from build123d import *

# Parameters (mm, degrees)
SKETCH1_R                       = 57.15
BOSS_EXTRUDE1_DEPTH             = 201.2442
SKETCH3_W                       = 1.27
SKETCH3_H                       = 1.27
SKETCH9_R                       = 61.1124
BOSS_EXTRUDE4_DEPTH             = 6.35
SKETCH10_R                      = 61.1124
BOSS_EXTRUDE5_DEPTH             = 6.35
F_97_0_164_DIAMETER_HOLE1_D     = 4.1656
F_97_0_164_DIAMETER_HOLE1_DEPTH = 8.255
F_97_0_164_DIAMETER_HOLE1_TIP   = 1.251472497
F_97_0_352_DIAMETER_HOLE1_D     = 8.9408
CUT_EXTRUDE3_DEPTH              = 202.2442
SKETCH20_R                      = 49.53
CUT_EXTRUDE4_DEPTH              = 191.7192
FILLET4_R                       = 0.508
FILLET5_R                       = 0.254
CHAMFER1_SIZE                   = 0.762
CHAMFER2_SIZE                   = 1.6002


with BuildPart() as part:
    # Sketch1 → Boss-Extrude1 (new body)
    with BuildSketch(Plane.XY):
        Circle(SKETCH1_R)
    extrude(amount=BOSS_EXTRUDE1_DEPTH)

    # Sketch3 → Cut-Revolve2 (revolve, cut)
    with BuildSketch(Plane(origin=(0, 0, 0), x_dir=(0, 0, -1), z_dir=(1, 0, 0))):
        with Locations((-31.115, 56.515)):
            Rectangle(SKETCH3_W, SKETCH3_H)
        with Locations((-189.357, 56.515)):
            Rectangle(SKETCH3_W, SKETCH3_H)
    revolve(axis=Axis((0, 0, 212.826037786), (0, 0, -1)), mode=Mode.SUBTRACT)

    # Sketch9 → Boss-Extrude4 (add)
    with BuildSketch(Plane.XY.offset(188.722)):
        Circle(SKETCH9_R)
    extrude(amount=-BOSS_EXTRUDE4_DEPTH)

    # Sketch10 → Boss-Extrude5 (add)
    with BuildSketch(Plane(origin=(0, 0, 31.75), x_dir=(-1, 0, 0), z_dir=(0, 0, -1))):
        Circle(SKETCH10_R)
    extrude(amount=-BOSS_EXTRUDE5_DEPTH)

    # #97 (0.164) Diameter Hole1
    with Locations(Plane.XY.offset(201.2442)):
        with Locations((0, 53.34), (46.193795038, 26.67), (46.193795038, -26.67), (0, -53.34), (-46.193795038, -26.67), (-46.193795038, 26.67)):
            Hole(F_97_0_164_DIAMETER_HOLE1_D / 2, depth=F_97_0_164_DIAMETER_HOLE1_DEPTH)
            with Locations((0, 0, -(F_97_0_164_DIAMETER_HOLE1_DEPTH + F_97_0_164_DIAMETER_HOLE1_TIP / 2))):  # 118° drill point
                Cone(0, F_97_0_164_DIAMETER_HOLE1_D / 2, F_97_0_164_DIAMETER_HOLE1_TIP, mode=Mode.SUBTRACT)

    # #97 (0.352) Diameter Hole1 (through all)
    with Locations(Plane.XY.offset(201.2442)):
        with Locations((0, 38.735), (33.545494016, 19.3675), (33.545494016, -19.3675), (0, -38.735), (-33.545494016, -19.3675), (-33.545494016, 19.3675)):
            Hole(F_97_0_352_DIAMETER_HOLE1_D / 2)

    # Sketch18 → Cut-Extrude3 (cut, through all)
    with BuildSketch(Plane.XY.offset(201.2442)):
        with BuildLine():
            Line((26.579810552, 10.4902), (32.11926165, 10.4902))
            ThreePointArc((32.11926165, 10.4902), (36.312562564, 8.908714176), (38.417156092, 4.952003922))
            ThreePointArc((38.417156092, 4.952003922), (38.655457352, 2.481096914), (38.735, 0))
            ThreePointArc((38.735, 0), (38.655457352, -2.481096914), (38.417156092, -4.952003922))
            ThreePointArc((38.417156092, -4.952003922), (36.312562564, -8.908714176), (32.11926165, -10.4902))
            Line((32.11926165, -10.4902), (26.579810552, -10.4902))
            ThreePointArc((26.579810552, -10.4902), (24.746675913, -14.2875), (22.374684967, -17.773691165))
            Line((22.374684967, -17.773691165), (25.144410516, -22.57099654))
            ThreePointArc((25.144410516, -22.57099654), (25.871454074, -26.993244568), (23.497139241, -30.794231156))
            ThreePointArc((23.497139241, -30.794231156), (21.476421633, -32.236059605), (19.3675, -33.545494016))
            ThreePointArc((19.3675, -33.545494016), (17.179035719, -34.717156519), (14.92001685, -35.746235077))
            ThreePointArc((14.92001685, -35.746235077), (10.44110849, -35.901958745), (6.974851134, -33.06119654))
            Line((6.974851134, -33.06119654), (4.205125585, -28.263891165))
            ThreePointArc((4.205125585, -28.263891165), (0, -28.575), (-4.205125585, -28.263891165))
            Line((-4.205125585, -28.263891165), (-6.974851134, -33.06119654))
            ThreePointArc((-6.974851134, -33.06119654), (-10.44110849, -35.901958745), (-14.92001685, -35.746235077))
            ThreePointArc((-14.92001685, -35.746235077), (-17.179035719, -34.717156519), (-19.3675, -33.545494016))
            ThreePointArc((-19.3675, -33.545494016), (-21.476421633, -32.236059605), (-23.497139241, -30.794231156))
            ThreePointArc((-23.497139241, -30.794231156), (-25.871454074, -26.993244568), (-25.144410516, -22.57099654))
            Line((-25.144410516, -22.57099654), (-22.374684967, -17.773691165))
            ThreePointArc((-22.374684967, -17.773691165), (-24.746675913, -14.2875), (-26.579810552, -10.4902))
            Line((-26.579810552, -10.4902), (-32.11926165, -10.4902))
            ThreePointArc((-32.11926165, -10.4902), (-36.312562564, -8.908714176), (-38.417156092, -4.952003922))
            ThreePointArc((-38.417156092, -4.952003922), (-38.655457352, -2.481096914), (-38.735, 0))
            ThreePointArc((-38.735, 0), (-38.655457352, 2.481096914), (-38.417156092, 4.952003922))
            ThreePointArc((-38.417156092, 4.952003922), (-36.312562564, 8.908714176), (-32.11926165, 10.4902))
            Line((-32.11926165, 10.4902), (-26.579810552, 10.4902))
            ThreePointArc((-26.579810552, 10.4902), (-24.746675913, 14.2875), (-22.374684967, 17.773691165))
            Line((-22.374684967, 17.773691165), (-25.144410516, 22.57099654))
            ThreePointArc((-25.144410516, 22.57099654), (-25.871454074, 26.993244568), (-23.497139241, 30.794231156))
            ThreePointArc((-23.497139241, 30.794231156), (-21.476421633, 32.236059605), (-19.3675, 33.545494016))
            ThreePointArc((-19.3675, 33.545494016), (-17.179035719, 34.717156519), (-14.92001685, 35.746235077))
            ThreePointArc((-14.92001685, 35.746235077), (-10.44110849, 35.901958745), (-6.974851134, 33.06119654))
            Line((-6.974851134, 33.06119654), (-4.205125585, 28.263891165))
            ThreePointArc((-4.205125585, 28.263891165), (0, 28.575), (4.205125585, 28.263891165))
            Line((4.205125585, 28.263891165), (6.974851134, 33.06119654))
            ThreePointArc((6.974851134, 33.06119654), (10.44110849, 35.901958745), (14.92001685, 35.746235077))
            ThreePointArc((14.92001685, 35.746235077), (17.179035719, 34.717156519), (19.3675, 33.545494016))
            ThreePointArc((19.3675, 33.545494016), (21.476421633, 32.236059605), (23.497139241, 30.794231156))
            ThreePointArc((23.497139241, 30.794231156), (25.871454074, 26.993244568), (25.144410516, 22.57099654))
            Line((25.144410516, 22.57099654), (22.374684967, 17.773691165))
            ThreePointArc((22.374684967, 17.773691165), (24.746675913, 14.2875), (26.579810552, 10.4902))
        make_face()
    extrude(amount=-CUT_EXTRUDE3_DEPTH, mode=Mode.SUBTRACT)

    # Sketch20 → Cut-Extrude4 (cut)
    with BuildSketch(Plane.XY.offset(201.2442)):
        Circle(SKETCH20_R)
    extrude(amount=-CUT_EXTRUDE4_DEPTH, mode=Mode.SUBTRACT)

    # Fillet4
    fillet4_edges = [part.edges().sort_by_distance(p)[0] for p in [
        (-49.53, 0, 9.525),
    ]]
    fillet(fillet4_edges, radius=FILLET4_R)

    # Fillet5
    fillet5_edges = [part.edges().sort_by_distance(p)[0] for p in [
        (-57.15, 0, 182.372),
        (-57.15, 0, 38.1),
    ]]
    fillet(fillet5_edges, radius=FILLET5_R)

    # Chamfer1
    chamfer1_edges = [part.edges().sort_by_distance(p)[0] for p in [
        (-57.15, 0, 201.2442),
    ]]
    chamfer(chamfer1_edges, length=CHAMFER1_SIZE)

    # Chamfer2
    chamfer2_edges = [part.edges().sort_by_distance(p)[0] for p in [
        (-57.15, 0, 0),
    ]]
    chamfer(chamfer2_edges, length=CHAMFER2_SIZE)


solid = part.part
Design review of the part built by this model. Coordinates are the model's own, in mm. A direction names the side the tool comes from. Give positions to 0.01 mm unless a question says otherwise; leave off trailing zeros. Order: outer loops, then holes, each group sorted by start corner. A loop starts at its lowest first (then second) coordinate and runs counter-clockwise, first axis right, second up.
1. Add section A-A, the plane z = 74.5. State the section outline as (x, y) points, then the cut area to 3 significant figures.
Solution:
outline: circle Ø114.3 at (0, 0); hole circle Ø99.06 at (0, 0)
area: 2,550 mm2
2. To check wall thickness, follow L1, parallel to Y at x = 0, z = 197.75; L2, parallel to Z at x = -52, y = 29.5; L3, parallel to X at y = -26.67, z = 195.5. State the ranges of each line that lie inside material, in increasing order.
Solution:
L1: y = -57.15 to -55.42, -51.26 to -49.53, 49.53 to 51.26, 55.42 to 57.15
L2: z = 31.75 to 38.1, 182.37 to 188.72
L3: x = -50.55 to -48.28, -44.11 to -41.74, 41.74 to 44.11, 48.28 to 50.55
3. Mouldability with a two-part tool opening along X and no side actions: class faces 4 (the flat face through (-55, -12, 30.48)), 5 (the cylindrical face through (0.582, 43.167, 4.696)), 6 (the conical face through (-0.078, -53.693, 191.955)), 7 (the cylindrical face through (54.5, 17.2, 15.8)) as +X half, -X half, draft (parallel to the pull), parting line (faces both ways), or undercut.
Solution:
face 4: draft
face 5: undercut
face 6: undercut
face 7: parting line
4. Add section B-B, the plane z = 34. State the section outline as (x, y) points.
Solution:
outline: circle Ø122.22 at (0, 0); hole circle Ø99.06 at (0, 0)
5. Tool access review of faces 1 (the cylindrical face through (-24.717, -14.339, 4.829)), 2 (the cylindrical face through (55.4, -7.3, 31.1)), 3 (the cylindrical face through (-48.118, -27.468, 197.059)): name each direction out of +Z, -Z, +X, -X, +Y, -Y from which nothing blocks a thin tool from reaching the whole face with its end or side.
Solution:
face 1: +Z, -Z
face 2: none
face 3: +Z
6. For pin 1 Ø3 at (x, z) = (29.5, 3) entering from -Y; pin 2 Ø4.5 at (x, z) = (30, 3.5) entering from +Y; pin 3 Ø10 at (y, z) = (-30, 20.5) entering from +X, all flat-tipped, find the tip position at first contact; note any pin that passes through.
Solution:
pin 1: stops at y = -49.82
pin 2: stops at y = 49.96
pin 3: stops at x = 51.39
